```python
from build123d import *

# Parameters (mm, degrees)
F0_W     = 304.8
F0_H     = 243.84
F0_R     = 2
F1_DEPTH = 1.6
F2_W     = 8.89
F2_H     = 84.84
F3_DEPTH = 11.25
F4_W     = 152.146
F4_H     = 28
F5_DEPTH = 37.338
F6_W     = 158.75
F6_H     = 44.45
F7_DEPTH = 1


with BuildPart() as f1:
    # F0 (on Top) → F1 (new body)
    with BuildSketch(Plane.XY):
        with Locations((152.4, 121.92)):
            Rectangle(F0_W, F0_H)
        with Locations((16.51, 6.35)):
            Circle(F0_R, mode=Mode.SUBTRACT)
        with Locations((140.97, 6.35)):
            Circle(F0_R, mode=Mode.SUBTRACT)
        with Locations((16.51, 78.74)):
            Circle(F0_R, mode=Mode.SUBTRACT)
        with Locations((140.97, 78.74)):
            Circle(F0_R, mode=Mode.SUBTRACT)
        with Locations((295.91, 6.35)):
            Circle(F0_R, mode=Mode.SUBTRACT)
        with Locations((295.91, 78.74)):
            Circle(F0_R, mode=Mode.SUBTRACT)
        with Locations((16.51, 233.68)):
            Circle(F0_R, mode=Mode.SUBTRACT)
        with Locations((95.25, 233.68)):
            Circle(F0_R, mode=Mode.SUBTRACT)
        with Locations((140.97, 233.68)):
            Circle(F0_R, mode=Mode.SUBTRACT)
        with Locations((295.91, 210.82)):
            Circle(F0_R, mode=Mode.SUBTRACT)
    extrude(amount=F1_DEPTH)

    # F2 (on face) → F3 (join)
    with BuildSketch(Plane.XY.offset(1.6)):
        with Locations((122.2248, 176.02)):
            Rectangle(F2_W, F2_H)
        with Locations((142.5448, 176.02)):
            Rectangle(F2_W, F2_H)
        with Locations((81.5848, 176.02)):
            Rectangle(F2_W, F2_H)
        with Locations((101.9048, 176.02)):
            Rectangle(F2_W, F2_H)
        with Locations((40.9448, 176.02)):
            Rectangle(F2_W, F2_H)
        with Locations((61.2648, 176.02)):
            Rectangle(F2_W, F2_H)
        with Locations((20.6248, 176.02)):
            Rectangle(F2_W, F2_H)
    extrude(amount=F3_DEPTH)

    # F4 (on face) → F5 (join)
    with BuildSketch(Plane.XY.offset(1.6)):
        with Locations((227.8634, 231.9482)):
            Rectangle(F4_W, F4_H)
    extrude(amount=F5_DEPTH)

    # F6 (on face) → F7 (join)
    with BuildSketch(Plane(origin=(0, 245.9482, 0), x_dir=(-1, 0, 0), z_dir=(0, 1, 0))):
        with Locations((-227.8634, 20.015)):
            Rectangle(F6_W, F6_H)
    extrude(amount=F7_DEPTH)


solid = f1.part
```
The listing builds one solid part. Answer for the finished solid, in the listing's coordinates (mm). A direction names the side the tool comes from. Round coordinates to 2 decimals unless told otherwise and drop trailing zeros. Order: outer loops, then holes, each group sorted by start corner. A loop starts at its lowest first (then second) coordinate and runs counter-clockwise, first axis right, second up. Notation, with made-up numbers: (-0.5, -30.5) - (4.5, -30.5) arc R29 ccw to (4.5, 3.5) - close; hole circle Ø1 at (39, 53.25). An arc over 180 degrees is marked (long way). Put each result on its own line as item: value. Start each with the question number.
(1) Find section C-C (x = 62.5). Give the vertices of the cut face in (y, z).
(2) Determine the mould class of faces 1 (the flat face through (142, 133.6, 7)), 2 (the flat face through (117.78, 175, 7)) for opening direction X: released by +X, released by -X, zero draft, split by the parting line, or undercut.
(3) Find section D-D (x = 238.5). Give the vertices of the cut face in (y, z), plus the area to 3 significant figures.
(4) Find section B-B (z = 33.5). Give the vertices of the cut face in (x, y).
(5) Straight lines are drawn through the part: probe 1 along Y at (x, z) = (16, 1); probe 2 along X at (y, z) = (233.68, 0.8); probe 3 along Y at (x, z) = (16.51, 0.75). For each, find the intervals that lie inside material, in ascending order. Write a range as from..to.
(6) Given P1, Ø3.5, axis at y = 191.5, z = 5, coming from the +X side; P2, Ø2, axis at x = 77.5, z = 12.5, coming from the -Y side; P3, Ø7, axis at x = 83, y = 169, coming from the +Z side, each flat-ended and moving along its own axis, determine where each tip first touches the part or whether it passes through.
(7) For faces 3 (the flat face through (41, 218.44, 7)), 4 (the flat face through (102, 133.6, 7)), 5 (the flat face through (150, 124, 0)), 6 (the flat face through (45.39, 175, 7)), determine the directions among +Z, -Z, +X, -X, +Y, -Y from which every point of the face is accessible in a straight line to the end or side of a thin tool.
Reply:
1. outline: (0, 0) - (243.84, 0) - (243.84, 1.6) - (218.44, 1.6) - (218.44, 12.85) - (133.6, 12.85) - (133.6, 1.6) - (0, 1.6) - close
2. face 1: zero draft
2. face 2: undercut
3. outline: (0, 0) - (243.84, 0) - (243.84, 1.6) - (245.95, 1.6) - (245.95, -2.21) - (246.95, -2.21) - (246.95, 42.24) - (245.95, 42.24) - (245.95, 38.94) - (217.95, 38.94) - (217.95, 1.6) - (0, 1.6) - close
3. area: 1,480 mm^2
4. outline: (148.49, 245.95) - (151.79, 245.95) - (151.79, 217.95) - (303.94, 217.95) - (303.94, 245.95) - (307.24, 245.95) - (307.24, 246.95) - (148.49, 246.95) - close
5. probe 1: 0..4.42, 8.28..76.81, 80.67..231.75, 235.61..243.84
5. probe 2: 0..14.51, 18.51..93.25, 97.25..138.97, 142.97..304.8
5. probe 3: 0..4.35, 8.35..76.74, 80.74..231.68, 235.68..243.84
6. P1: x = 146.99
6. P2: y = 133.6
6. P3: z = 12.85
7. face 3: +Z, -X, +Y
7. face 4: +Z, +X, -X, -Y
7. face 5: -Z, +X, -X, -Y
7. face 6: +Z, +Y, -Y
